Source: CAD feature listing. Evaluate the final solid. Frame: model axes, mm. Face numbers are marked on the shaded views. Round coordinates to 2 decimals unless told otherwise and drop trailing zeros. Write each loop counter-clockwise with the first axis right and the second up, starting at its lowest first coordinate (ties: lowest second). Pieces come first, ordered by that corner, then holes. Notation, with made-up numbers: M 85,-7 L 89,-7 A28 cw 89,11 Z; hole C -7.75,34.5 d9. An arc over 180 degrees is marked long. Answer in a Markdown table with one row per item.
from build123d import *

# Parameters (mm, degrees)
F3_DEPTH = 25.4


with BuildPart() as f1:
    # F0 (on Front) → F1 (revolve)
    with BuildSketch(Plane.XZ):
        Polygon((-38.1, 101.6), (0, 101.6), (0, 139.7), (-3.175, 139.7), (-3.175, 104.775), (-38.1, 104.775), align=None)
    revolve(axis=Axis((-40.6781, 0, 0), (-1, 0, 0)))

    # F2 (on Right) → F3 (cut)
    with BuildSketch(Plane.YZ):
        with BuildLine():
            Line((-110.5365962259, 63.8183335863), (-106.4121502404, 61.4370835863))
            ThreePointArc((-106.4121502404, 61.4370835863), (-105.201540854, 63.4877685883), (-103.951417404, 65.5146073641))
            ThreePointArc((-103.951417404, 65.5146073641), (-107.6001407887, 66.0490337928), (-110.5365962259, 63.8183335863))
        make_face()
        with BuildLine():
            ThreePointArc((-108.7130229983, 57.2672645493), (-107.582790854, 59.3633226027), (-106.4121502404, 61.4370835863))
            Line((-106.4121502404, 61.4370835863), (-110.5365962259, 63.8183335863))
            ThreePointArc((-110.5365962259, 63.8183335863), (-111.0002115544, 60.1599384774), (-108.7130229983, 57.2672645493))
        make_face()
        with BuildLine():
            ThreePointArc((-108.7130229983, 57.2672645493), (-105.1350051315, 56.8490222724), (-102.2877042549, 59.0558335863))
            Line((-102.2877042549, 59.0558335863), (-106.4121502404, 61.4370835863))
            ThreePointArc((-106.4121502404, 61.4370835863), (-107.582790854, 59.3633226027), (-108.7130229983, 57.2672645493))
        make_face()
        with BuildLine():
            Line((-106.4121502404, 61.4370835863), (-102.2877042549, 59.0558335863))
            ThreePointArc((-102.2877042549, 59.0558335863), (-101.8119284927, 60.204457884), (-101.6496502404, 61.4370835863))
            ThreePointArc((-101.6496502404, 61.4370835863), (-102.2648230057, 63.7782548869), (-103.951417404, 65.5146073641))
            ThreePointArc((-103.951417404, 65.5146073641), (-105.201540854, 63.4877685883), (-106.4121502404, 61.4370835863))
        make_face()
        with BuildLine():
            Line((-110.5365962259, -63.8183335863), (-106.4121502404, -61.4370835863))
            ThreePointArc((-106.4121502404, -61.4370835863), (-107.582790854, -59.3633226027), (-108.7130229983, -57.2672645493))
            ThreePointArc((-108.7130229983, -57.2672645493), (-111.0002115544, -60.1599384774), (-110.5365962259, -63.8183335863))
        make_face()
        with BuildLine():
            Line((-106.4121502404, -61.4370835863), (-102.2877042549, -59.0558335863))
            ThreePointArc((-102.2877042549, -59.0558335863), (-105.1350051315, -56.8490222724), (-108.7130229983, -57.2672645493))
            ThreePointArc((-108.7130229983, -57.2672645493), (-107.582790854, -59.3633226027), (-106.4121502404, -61.4370835863))
        make_face()
        with BuildLine():
            ThreePointArc((-101.6496502404, -61.4370835863), (-101.8119284927, -60.204457884), (-102.2877042549, -59.0558335863))
            Line((-102.2877042549, -59.0558335863), (-106.4121502404, -61.4370835863))
            ThreePointArc((-106.4121502404, -61.4370835863), (-105.201540854, -63.4877685883), (-103.951417404, -65.5146073641))
            ThreePointArc((-103.951417404, -65.5146073641), (-102.2648230057, -63.7782548869), (-101.6496502404, -61.4370835863))
        make_face()
        with BuildLine():
            ThreePointArc((-103.951417404, -65.5146073641), (-105.201540854, -63.4877685883), (-106.4121502404, -61.4370835863))
            Line((-106.4121502404, -61.4370835863), (-110.5365962259, -63.8183335863))
            ThreePointArc((-110.5365962259, -63.8183335863), (-107.6001407887, -66.0490337928), (-103.951417404, -65.5146073641))
        make_face()
        with BuildLine():
            ThreePointArc((4.7625, -122.8741671727), (4.7622763933, -122.8280173762), (4.7616055942, -122.7818719133))
            ThreePointArc((4.7616055942, -122.7818719133), (2.38125, -122.851091191), (0, -122.8741671727))
            Line((0, -122.8741671727), (0, -127.6366671727))
            ThreePointArc((0, -127.6366671727), (3.3675960454, -126.2417632181), (4.7625, -122.8741671727))
        make_face()
        with BuildLine():
            ThreePointArc((4.7616055942, -122.7818719133), (3.3348050976, -119.474096407), (0, -118.1116671727))
            Line((0, -118.1116671727), (0, -122.8741671727))
            ThreePointArc((0, -122.8741671727), (2.38125, -122.851091191), (4.7616055942, -122.7818719133))
        make_face()
        with BuildLine():
            Line((0, -122.8741671727), (0, -118.1116671727))
            ThreePointArc((0, -118.1116671727), (-3.3348050976, -119.474096407), (-4.7616055942, -122.7818719133))
            ThreePointArc((-4.7616055942, -122.7818719133), (-2.38125, -122.851091191), (0, -122.8741671727))
        make_face()
        with BuildLine():
            Line((0, -127.6366671727), (0, -122.8741671727))
            ThreePointArc((0, -122.8741671727), (-2.38125, -122.851091191), (-4.7616055942, -122.7818719133))
            ThreePointArc((-4.7616055942, -122.7818719133), (-3.4000707656, -126.2089722702), (0, -127.6366671727))
        make_face()
        with BuildLine():
            ThreePointArc((106.4121502404, -61.4370835863), (107.582790854, -59.3633226027), (108.7130229983, -57.2672645493))
            ThreePointArc((108.7130229983, -57.2672645493), (105.1350051315, -56.8490222724), (102.2877042549, -59.0558335863))
            Line((102.2877042549, -59.0558335863), (106.4121502404, -61.4370835863))
        make_face()
        with BuildLine():
            ThreePointArc((111.1746502404, -61.4370835863), (110.5133276786, -59.0159784936), (108.7130229983, -57.2672645493))
            ThreePointArc((108.7130229983, -57.2672645493), (107.582790854, -59.3633226027), (106.4121502404, -61.4370835863))
            Line((106.4121502404, -61.4370835863), (110.5365962259, -63.8183335863))
            ThreePointArc((110.5365962259, -63.8183335863), (111.0123719881, -62.6697092886), (111.1746502404, -61.4370835863))
        make_face()
        with BuildLine():
            Line((110.5365962259, -63.8183335863), (106.4121502404, -61.4370835863))
            ThreePointArc((106.4121502404, -61.4370835863), (105.201540854, -63.4877685883), (103.951417404, -65.5146073641))
            ThreePointArc((103.951417404, -65.5146073641), (107.6001407887, -66.0490337928), (110.5365962259, -63.8183335863))
        make_face()
        with BuildLine():
            ThreePointArc((103.951417404, -65.5146073641), (105.201540854, -63.4877685883), (106.4121502404, -61.4370835863))
            Line((106.4121502404, -61.4370835863), (102.2877042549, -59.0558335863))
            ThreePointArc((102.2877042549, -59.0558335863), (101.8002000339, -62.6250741347), (103.951417404, -65.5146073641))
        make_face()
        with BuildLine():
            ThreePointArc((103.951417404, 65.5146073641), (105.201540854, 63.4877685883), (106.4121502404, 61.4370835863))
            Line((106.4121502404, 61.4370835863), (110.5365962259, 63.8183335863))
            ThreePointArc((110.5365962259, 63.8183335863), (107.6001407887, 66.0490337928), (103.951417404, 65.5146073641))
        make_face()
        with BuildLine():
            ThreePointArc((106.4121502404, 61.4370835863), (107.582790854, 59.3633226027), (108.7130229983, 57.2672645493))
            ThreePointArc((108.7130229983, 57.2672645493), (110.5133276786, 59.0159784936), (111.1746502404, 61.4370835863))
            ThreePointArc((111.1746502404, 61.4370835863), (111.0123719881, 62.6697092886), (110.5365962259, 63.8183335863))
            Line((110.5365962259, 63.8183335863), (106.4121502404, 61.4370835863))
        make_face()
        with BuildLine():
            ThreePointArc((102.2877042549, 59.0558335863), (105.1350051315, 56.8490222724), (108.7130229983, 57.2672645493))
            ThreePointArc((108.7130229983, 57.2672645493), (107.582790854, 59.3633226027), (106.4121502404, 61.4370835863))
            Line((106.4121502404, 61.4370835863), (102.2877042549, 59.0558335863))
        make_face()
        with BuildLine():
            Line((102.2877042549, 59.0558335863), (106.4121502404, 61.4370835863))
            ThreePointArc((106.4121502404, 61.4370835863), (105.201540854, 63.4877685883), (103.951417404, 65.5146073641))
            ThreePointArc((103.951417404, 65.5146073641), (101.8002000339, 62.6250741347), (102.2877042549, 59.0558335863))
        make_face()
        with BuildLine():
            ThreePointArc((0, 122.8741671727), (2.38125, 122.851091191), (4.7616055942, 122.7818719133))
            ThreePointArc((4.7616055942, 122.7818719133), (4.7622763933, 122.8280173762), (4.7625, 122.8741671727))
            ThreePointArc((4.7625, 122.8741671727), (3.3675960454, 126.2417632181), (0, 127.6366671727))
            Line((0, 127.6366671727), (0, 122.8741671727))
        make_face()
        with BuildLine():
            ThreePointArc((-4.7616055942, 122.7818719133), (-2.38125, 122.851091191), (0, 122.8741671727))
            Line((0, 122.8741671727), (0, 127.6366671727))
            ThreePointArc((0, 127.6366671727), (-3.4000707656, 126.2089722702), (-4.7616055942, 122.7818719133))
        make_face()
        with BuildLine():
            ThreePointArc((-4.7616055942, 122.7818719133), (-3.3348050976, 119.474096407), (0, 118.1116671727))
            Line((0, 118.1116671727), (0, 122.8741671727))
            ThreePointArc((0, 122.8741671727), (-2.38125, 122.851091191), (-4.7616055942, 122.7818719133))
        make_face()
        with BuildLine():
            ThreePointArc((0, 118.1116671727), (3.3348050976, 119.474096407), (4.7616055942, 122.7818719133))
            ThreePointArc((4.7616055942, 122.7818719133), (2.38125, 122.851091191), (0, 122.8741671727))
            Line((0, 122.8741671727), (0, 118.1116671727))
        make_face()
    extrude(amount=-F3_DEPTH, mode=Mode.SUBTRACT)


solid = f1.part
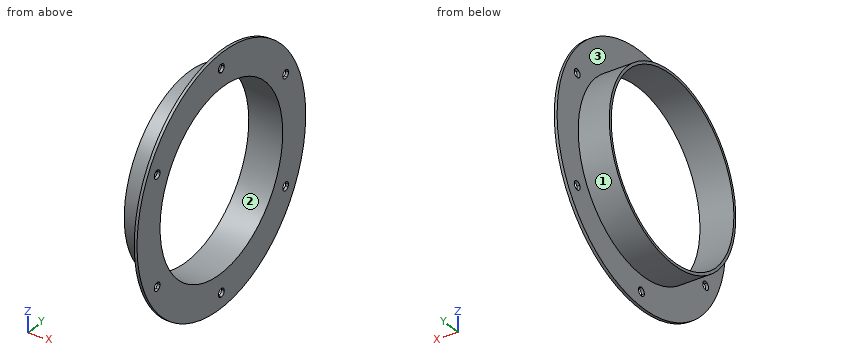
Q1. Section B-B (x = -13.5). Return loops of the section in (y, z) (3 decimals).
Solutions:
| item | result |
|---|---|
| outline | C 0,0 d209.55; hole C 0,0 d203.2 |
Q2. Contact query for flat-ended pins moving along their axis: pin 1 Ø12 at (x, z) = (-20, -72.5) entering from +Y; pin 2 Ø12 at (y, z) = (-56.5, 73) entering from +X; pin 3 Ø8 at (x, y) = (-21.5, -71.5) entering from -Z; pin 4 Ø4 at (x, z) = (-26.5, 63.5) entering from -Y. Output: stop coordinate, or through.
Solutions:
| item | result |
|---|---|
| pin 1 | stops at y = 80.97 |
| pin 2 | passes through |
| pin 3 | stops at z = -80.13 |
| pin 4 | stops at y = -84.83 |
Q3. Section C-C (y = -91). Return loops of the section in (x, z) (3 decimals), and give its area (3 significant figures).
Solutions:
| item | result |
|---|---|
| outline | M -38.1,-51.931 L -3.175,-51.931 L -3.175,-105.996 L 0,-105.996 L 0,-45.184 L -38.1,-45.184 Z; M -38.1,45.184 L 0,45.184 L 0,105.996 L -3.175,105.996 L -3.175,51.931 L -38.1,51.931 Z |
| area | 857 mm2 |
Q4. Material intervals for probe 1 along Y at (x, z) = (-12.5, 0) (3 decimals); probe 2 along Z at (x, y) = (-25, -58); probe 3 along Y at (x, z) = (-26, 63), sorted ascending.
Solutions:
| item | result |
|---|---|
| probe 1 | y = -104.775 to -101.6, 101.6 to 104.775 |
| probe 2 | z = -87.26 to -83.42, 83.42 to 87.26 |
| probe 3 | y = -83.72 to -79.71, 79.71 to 83.72 |
Q5. Pull-direction query (Z, two-part tool) for the marked faces 1, 2 and 3; classes: pulls with the +Z half, pulls with the -Z half, needs draft (parallel to the pull), parting line crosses it, or undercut.
Solutions:
| item | result |
|---|---|
| face 1 | parting line crosses it |
| face 2 | undercut |
| face 3 | needs draft |
Q6. Section A-A (z = 0). Return loops of the section in (x, y) (3 decimals).
Solutions:
| item | result |
|---|---|
| outline | M -38.1,-104.775 L -3.175,-104.775 L -3.175,-139.7 L 0,-139.7 L 0,-101.6 L -38.1,-101.6 Z; M -38.1,101.6 L 0,101.6 L 0,139.7 L -3.175,139.7 L -3.175,104.775 L -38.1,104.775 Z |
Q7. Section D-D (y = -120). Return loops of the section in (x, z) (3 decimals), and give its area (3 significant figures).
Solutions:
| item | result |
|---|---|
| outline | M -3.175,-71.527 L 0,-71.527 L 0,71.527 L -3.175,71.527 Z |
| area | 454 mm2 |
